Check sheet for the drawn part. Datum: minimum x, y, z corner. Units: mm. A direction names the side the tool comes from. Give positions to 0.01 mm unless a question says otherwise; leave off trailing zeros. Order: outer loops, then holes, each group sorted by start corner. A loop starts at its lowest first (then second) coordinate and runs counter-clockwise, first axis right, second up. Notation, with made-up numbers: M 73.5,-2.75 L 83.5,-2.75 A25 cw 83.5,32.25 Z; hole C 11,-16.75 d7. An arc over 180 degrees is marked long. Put each result on its own line as item: value. Start each with the question number.
Q1. Material ranges on L1, parallel to Z at x = 15.5, y = 59.89; L2, parallel to Y at x = 9, z = 5.25; L3, parallel to Y at x = 11, z = 1 (1 decimal), recorded low to high.
Q2. Section check B-B on z = 6.6. Record the cut outline in (x, y).
Q3. Section check D-D on y = 5. Record the cut outline in (x, z), then the cut area to 3 significant figures.
Q4. Access from +Z, -Z, +X, -X, +Y, -Y to the whole of each face (thin tool, end or side, straight path). Record for the marked faces 1, 2 and 3.
Q5. Section check A-A on y = 59.89. Record the cut outline in (x, z).
Q6. Go/stop test with flat-tipped pins: pin 1 (4 mm diameter, centred on x = 19.5, z = 6.5, fed in from -Y); pin 2 (3.5 mm diameter, centred on x = 3, z = 4, fed in from +Y); pin 3 (2 mm diameter, centred on y = 60, z = 6, fed in from -X); pin 4 (6 mm diameter, centred on x = 22.5, y = 30.5, fed in from +Z). Record where each tip stops, or that it passes through.
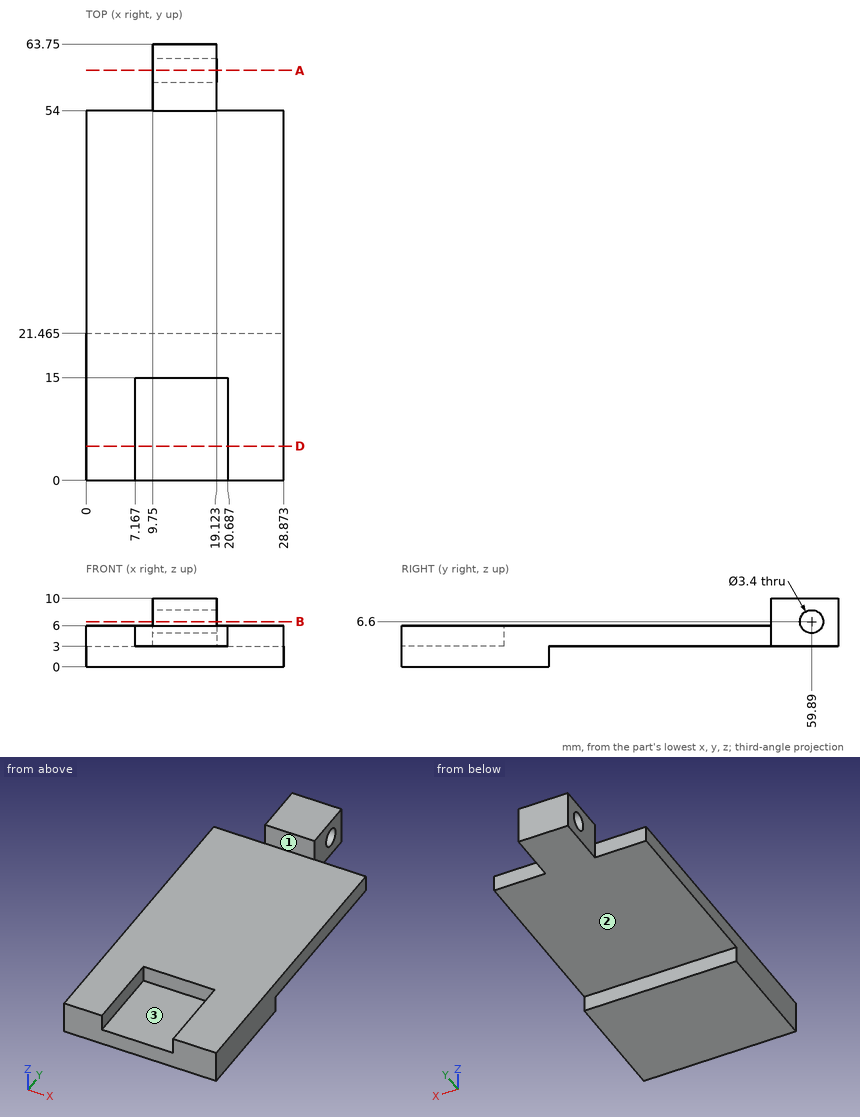
Results found:
1. L1: z = 3 to 4.9, 8.3 to 10
1. L2: y = 15 to 54
1. L3: y = 0 to 21.5
2. outline: M 9.75,54 L 19.12,54 L 19.12,58.19 L 9.75,58.19 Z; M 9.75,61.59 L 19.12,61.59 L 19.12,63.75 L 9.75,63.75 Z
3. outline: M 0,0 L 28.87,0 L 28.87,6 L 20.69,6 L 20.69,3 L 7.17,3 L 7.17,6 L 0,6 Z
3. area: 133 mm^2
4. face 1: +Z, +X, -X, -Y
4. face 2: -Z, +X, -X, +Y
4. face 3: +Z, -Y
5. outline: M 9.75,3 L 19.12,3 L 19.12,4.9 L 9.75,4.9 Z; M 9.75,8.3 L 19.12,8.3 L 19.12,10 L 9.75,10 Z
6. pin 1: stops at y = 0
6. pin 2: stops at y = 54
6. pin 3: passes through
6. pin 4: stops at z = 6
